Source: three-view drawing plus pictorial views. Frame: mm from the lowest corner of the part. A direction names the side the tool comes from. Give positions to 0.01 mm unless a question says otherwise; leave off trailing zeros. Loops run counter-clockwise (first coordinate to the right, second up) from the corner with the lowest first, then second, coordinate; pieces in that order, holes last. Notation, with made-up numbers: (1.5, 20) - (48.5, 20) arc R20 cw to (48.5, 51) - close; hole circle Ø1 at (44, -33). An arc over 180 degrees is marked (long way). Answer in a Markdown table with one row per item.
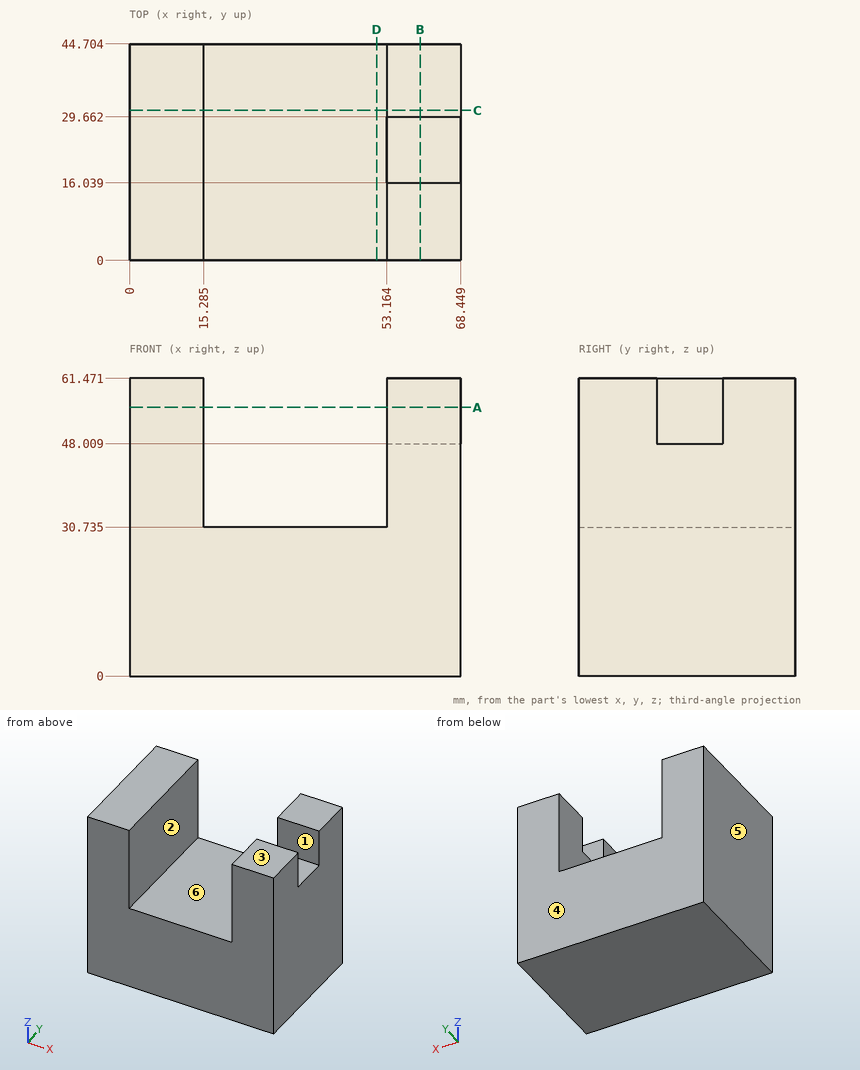
Q1. Draft query along X for the marked faces 4, 5 and 6. Return one class per face: pulls with the +X half, pulls with the -X half, needs draft (parallel to the pull), parting line crosses it, or undercut.
Check values:
| item | result |
|---|---|
| face 4 | needs draft |
| face 5 | pulls with the -X half |
| face 6 | undercut |
Q2. Material intervals for line 1 along X through (y, z) = (31, 42) (1 decimal); line 2 along Y through (x, z) = (56.5, 54); line 3 along Z through (x, y) = (45.5, 21) (1 decimal), sorted ascending.
Check values:
| item | result |
|---|---|
| line 1 | 0 to 15.3, 53.2 to 68.4 |
| line 2 | 0 to 16.04, 29.66 to 44.7 |
| line 3 | 0 to 30.7 |
Q3. Reachability of the marked faces 1, 2 and 3 from +Z, -Z, +X, -X, +Y, -Y: full face, straight path, thin tool, end or side. Return the list, or none.
Check values:
| item | result |
|---|---|
| face 1 | +Z, +X |
| face 2 | +Z, +Y, -Y |
| face 3 | +Z, +X, -X, +Y, -Y |
Q4. First-contact query: pin 1 (11 mm diameter, centred on x = 64, y = 23.5, fed in from +Z); pin 2 (19 mm diameter, centred on x = 25.5, y = 14.5, fed in from +Z) (1 decimal). Flat tips, straight axial feed; report the tip coordinate or a pass-through.
Check values:
| item | result |
|---|---|
| pin 1 | z = 48.01 |
| pin 2 | z = 30.7 |
Q5. Cut plane C-C (y = 31). Output: boundary loops of the cut face in (x, z) (1 decimal), and give its area (3 significant figures).
Check values:
| item | result |
|---|---|
| outline | (0, 0) - (68.4, 0) - (68.4, 61.5) - (53.2, 61.5) - (53.2, 30.7) - (15.3, 30.7) - (15.3, 61.5) - (0, 61.5) - close |
| area | 3,040 mm² |
Q6. Cut plane B-B (x = 60). Output: boundary loops of the cut face in (y, z), and give its area (3 significant figures).
Check values:
| item | result |
|---|---|
| outline | (0, 0) - (44.7, 0) - (44.7, 61.47) - (29.66, 61.47) - (29.66, 48.01) - (16.04, 48.01) - (16.04, 61.47) - (0, 61.47) - close |
| area | 2,560 mm² |
Q7. Cut plane D-D (x = 51). Output: boundary loops of the cut face in (y, z) (1 decimal), and give its area (3 significant figures).
Check values:
| item | result |
|---|---|
| outline | (0, 0) - (44.7, 0) - (44.7, 30.7) - (0, 30.7) - close |
| area | 1,370 mm² |
Q8. Cut plane A-A (z = 55.5). Output: boundary loops of the cut face in (x, y) (1 decimal).
Check values:
| item | result |
|---|---|
| outline | (0, 0) - (15.3, 0) - (15.3, 44.7) - (0, 44.7) - close; (53.2, 0) - (68.4, 0) - (68.4, 16) - (53.2, 16) - close; (53.2, 29.7) - (68.4, 29.7) - (68.4, 44.7) - (53.2, 44.7) - close |
